Part model, mm, in its own coordinate system. A direction names the side the tool comes from. Round coordinates to 2 decimals unless told otherwise and drop trailing zeros. Write each loop counter-clockwise with the first axis right and the second up, starting at its lowest first coordinate (ties: lowest second). Pieces come first, ordered by that corner, then holes. Notation, with made-up numbers: (-13, 42.25) -> (45, 42.25) arc R32 cw to (45, 69.25) -> close; hole circle Ø6 at (-9, 47). An arc over 180 degrees is marked (long way). Return JSON: item names as keys, results as strings. Group by question number.
```python
from build123d import *

# Parameters (mm, degrees)
F0_R      = 5
F1_DEPTH  = 30
F1_FACE_R = 5
F3_ANGLE  = 90
F4_DEPTH  = 120


with BuildPart() as f1:
    # F0 (on Front) → F1 (new body)
    with BuildSketch(Plane.XZ):
        Circle(F0_R)
    extrude(amount=F1_DEPTH)

    # F1_face (on face) → F3 (revolve)
    with BuildSketch(Plane(origin=(0, 0, 0), x_dir=(1, 0, 0), z_dir=(0, 1, 0))):
        Circle(F1_FACE_R)
    revolve(axis=Axis((-10.6502734125, 0, 14.0971038491), (1, 0, 0)), revolution_arc=F3_ANGLE)

    # F4 (add): a face of the model
    f4_faces = [f1.faces().sort_by_distance(p)[0] for p in [
        (0, 14.0971038491, 14.0971038491),
    ]]
    extrude(f4_faces, amount=F4_DEPTH)


solid = f1.part
```
Item 1: Cut at A-A (x = 0). Write the cut outline in (y, z), then the cut area to 3 significant figures.
Item 2: Wall check: L1, parallel to Z at x = -0.25, y = -15.5; L2, parallel to Y at x = -0.5, z = 103.5; L3, parallel to X at y = 15, z = 15. Give the ranges that are in metal, low to high.
Item 3: Cut at B-B (z = 92). Write the cut outline in (x, y).
Item 4: Cut at C-C (y = -10.5). Write the cut outline in (x, z), then the cut area to 3 significant figures.
Item 5: Which spindle directions (+Z, -Z, +X, -X, +Y, -Y) get a long thin tool onto all of the face, cutting with end or side? Do faces 1 (the face through (-1.084, 9.216, 73.257)), 2 (the face through (0, 14, 134.097)), 3 (the face through (-1.08, -14.79, -4.88)). Say none if no direction does.
Item 6: Flat gauge pins, fed straight in: P1, Ø5, axis at x = 0.5, y = -5.5, coming from the -Z side; P2, Ø8, axis at y = 3.5, z = 116.5, coming from the -X side. Where does each tip first touch, or does it go through?
Checks:
{
 "1": {"outline": "(-30, -5) -> (0, -5) arc R19.1 ccw to (19.1, 14.1) -> (19.1, 134.1) -> (9.1, 134.1) -> (9.1, 14.1) arc R9.1 cw to (0, 5) -> (-30, 5) -> close", "area": "1,720 mm2"},
 "2": {"L1": "z = -4.99 to 4.99", "L2": "y = 9.12 to 19.07", "L3": "x = -4.92 to 4.92"},
 "3": {"outline": "circle Ø10 at (0, 14.1)"},
 "4": {"outline": "circle Ø10 at (0, 0)", "area": "78.5 mm2"},
 "5": {"face 1": "+Z", "face 2": "+Z, +X, -X, +Y, -Y", "face 3": "-Y"},
 "6": {"P1": "stops at z = -5", "P2": "passes through"}
}
